Answer from the drawing. Dimensions are ordinates in mm from the lowest x, y and z of the part. Coordinates: 2 decimals unless noted, no trailing zeros. Order: outer loops, then holes, each group sorted by start corner. A loop starts at its lowest first (then second) coordinate and runs counter-clockwise, first axis right, second up. Notation, with made-up numbers: (-17, 59.25) - (38, 59.25) arc R20 ccw to (38, 84.25) - close; hole circle Ø7 at (40.25, 15.5). An arc over 180 degrees is marked (long way). Use a Markdown table: item, result. Add a question column.
Item 1: Find the intervals of material crossed by line 1 along Z through (x, y) = (8, 3.5); line 2 along X through (y, z) = (10.5, 8.75); line 3 along Z through (x, y) = (5, 2.5), in increasing order.
Item 2: The part is cut by section A-A, the plane y = 2.75. Give the vertices of the cut face in (x, z), then the cut area to 3 significant figures.
Item 3: Flat-ended cylindrical pins translate along their axes: P1, Ø5, axis at x = 9, z = 7.5, coming from the -Y side; P2, Ø4, axis at x = 14, y = 5.5, coming from the -Z side; P3, Ø1.5, axis at y = 9.5, z = 5.5, coming from the -X side; P4, Ø4, axis at x = 8, z = 8, coming from the +Y side. Find the tip coordinate at first contact, or state that the pin passes through.
Item 4: The mould has two halves that part along X. Classify the marked faces 1, 2 and 3: released by +X, released by -X, zero draft, split by the parting line, or undercut.
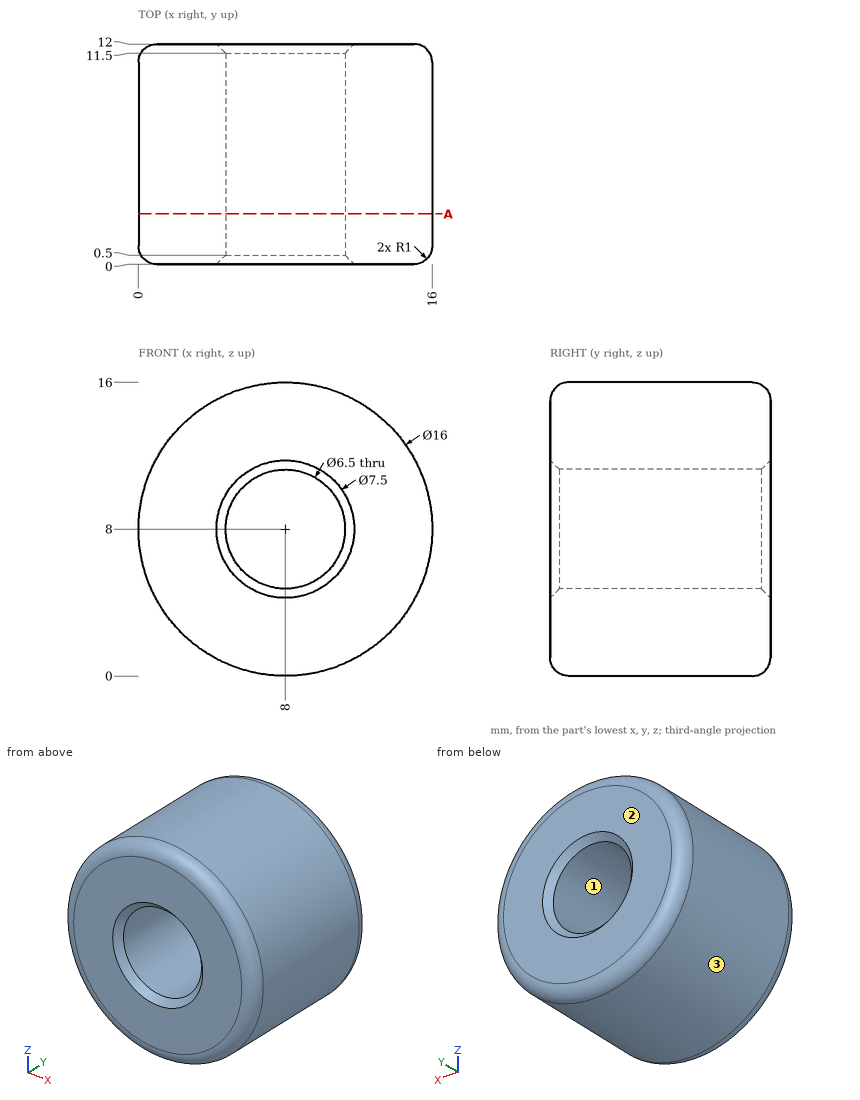
Solution:
| question | item | result |
|---|---|---|
| 1 | line 1 | z = 0 to 4.75, 11.25 to 16 |
| 1 | line 2 | x = 0.04 to 4.84, 11.16 to 15.96 |
| 1 | line 3 | z = 0.58 to 6.75, 9.25 to 15.42 |
| 2 | outline | circle Ø16 at (8, 8); hole circle Ø6.5 at (8, 8) |
| 2 | area | 168 mm2 |
| 3 | P1 | stops at y = 0.13 |
| 3 | P2 | stops at z = 1.07 |
| 3 | P3 | stops at x = 0.19 |
| 3 | P4 | passes through |
| 4 | face 1 | undercut |
| 4 | face 2 | zero draft |
| 4 | face 3 | split by the parting line |
